Could you check a few things on this drawing? It's one solid part, dimensions in mm from its lowest x, y, z. A direction names the side the tool comes from. Give positions to 0.01 mm unless a question says otherwise; leave off trailing zeros. Loops run counter-clockwise (first coordinate to the right, second up) from the corner with the lowest first, then second, coordinate; pieces in that order, holes last.
1. Imagine slicing it at D-D (z = 3). List the corners of the cut face in (x, y) for me.
2. For the marked faces 1, 2, 3 and 4, which set-ups out of +Z, -Z, +X, -X, +Y, -Y let a thin tool reach every point of the face, with its end or its side?
3. Imagine slicing it at B-B (y = 13.25). List the corners of the cut face in (x, z) for me.
4. For P1, Ø6.5, axis at x = 86, z = 29, coming from the +Y side; P2, Ø1.5, axis at y = 5.5, z = 9.5, coming from the -X side; P3, Ø6, axis at x = 38.5, y = 20.5, coming from the +Z side; P4, Ø6.5, axis at y = 9.5, z = 20, coming from the +X side, each with a flat end and sliding along its axis, tell me the tip position at first contact or that it passes through.
5. Imagine slicing it at A-A (z = 20). List the corners of the cut face in (x, y) for me, plus the area to 3 significant figures.
6. Imagine slicing it at C-C (x = 50.75). List the corners of the cut face in (y, z) for me, plus the area to 3 significant figures.
7. Thinking about a two-plate mould opening in X: for the marked faces 5, 6 and 7, which applies, +X half, -X half, draft (parallel to the pull), parting line (faces both ways), or undercut?
8. I need wall thicknesses on line 1 along X through (y, z) = (8, 3); line 2 along X through (y, z) = (26.1, 20); line 3 along Y through (x, z) = (93, 22). Which ranges of each line are inside material? Lowest first, please.
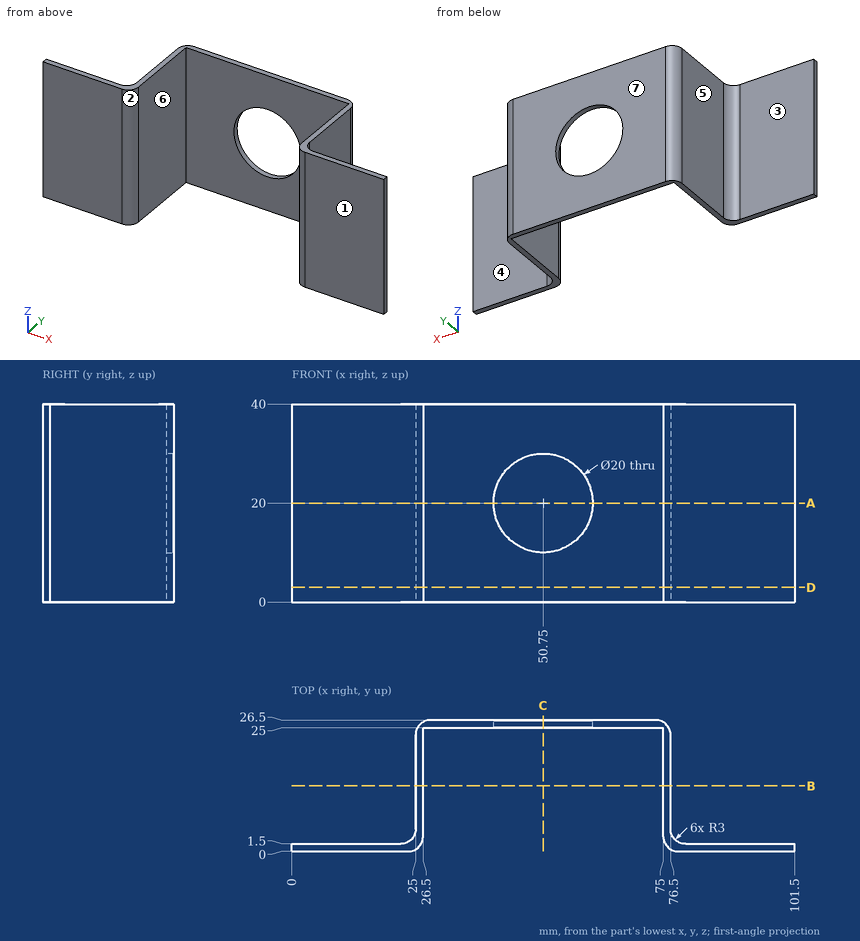
Derived:
1. outline: (0, 0) - (23.5, 0) arc R3 ccw to (26.5, 3) - (26.5, 25) - (75, 25) - (75, 3) arc R3 ccw to (78, 0) - (101.5, 0) - (101.5, 1.5) - (79.5, 1.5) arc R3 cw to (76.5, 4.5) - (76.5, 23.5) arc R3 ccw to (73.5, 26.5) - (28, 26.5) arc R3 ccw to (25, 23.5) - (25, 4.5) arc R3 cw to (22, 1.5) - (0, 1.5) - close
2. face 1: +Z, -Z, +X, -X, -Y
2. face 2: +Z, -Z, -Y
2. face 3: +Z, -Z, -X, +Y
2. face 4: +Z, -Z, +X, +Y
3. outline: (25, 0) - (26.5, 0) - (26.5, 40) - (25, 40) - close; (75, 0) - (76.5, 0) - (76.5, 40) - (75, 40) - close
4. P1: stops at y = 1.5
4. P2: stops at x = 25
4. P3: passes through
4. P4: stops at x = 76.5
5. outline: (0, 0) - (23.5, 0) arc R3 ccw to (26.5, 3) - (26.5, 25) - (40.75, 25) - (40.75, 26.5) - (28, 26.5) arc R3 ccw to (25, 23.5) - (25, 4.5) arc R3 cw to (22, 1.5) - (0, 1.5) - close; (60.75, 25) - (75, 25) - (75, 3) arc R3 ccw to (78, 0) - (101.5, 0) - (101.5, 1.5) - (79.5, 1.5) arc R3 cw to (76.5, 4.5) - (76.5, 23.5) arc R3 ccw to (73.5, 26.5) - (60.75, 26.5) - close
5. area: 193 mm2
6. outline: (25, 0) - (26.5, 0) - (26.5, 10) - (25, 10) - close; (25, 30) - (26.5, 30) - (26.5, 40) - (25, 40) - close
6. area: 30.0 mm2
7. face 5: -X half
7. face 6: undercut
7. face 7: draft
8. line 1: x = 25 to 26.5, 75 to 76.5
8. line 2: x = 26.5 to 40.75, 60.75 to 75
8. line 3: y = 0 to 1.5
